```python
from build123d import *

# Parameters (mm, degrees)
EXTRUDE_1_DEPTH     = 1
EXTRUDE_2_DEPTH     = 20
CUT_EXTRUDE_1_DEPTH = 20


with BuildPart() as part:
    # 草图1 → 凸台-拉伸1 (new body)
    with BuildSketch(Plane.XY):
        with BuildLine():
            Line((0, 38), (33, 38))
            ThreePointArc((33, 38), (71, 0), (33, -38))
            Line((33, -38), (0, -38))
            ThreePointArc((0, -38), (-38, 0), (0, 38))
        make_face()
    extrude(amount=EXTRUDE_1_DEPTH)

    # 草图2 → 凸台-拉伸2 (add)
    with BuildSketch(Plane.XY.offset(1)):
        with BuildLine():
            Line((0, 38), (33, 38))
            ThreePointArc((33, 38), (71, 0), (33, -38))
            Line((33, -38), (0, -38))
            ThreePointArc((0, -38), (-38, 0), (0, 38))
        make_face()
        with BuildLine():
            Line((0, 37), (33, 37))
            ThreePointArc((33, 37), (70, 0), (33, -37))
            Line((33, -37), (0, -37))
            ThreePointArc((0, -37), (-37, 0), (0, 37))
        make_face(mode=Mode.SUBTRACT)
    extrude(amount=EXTRUDE_2_DEPTH)

    # 草图3 → 切除-拉伸1 (cut)
    with BuildSketch(Plane.XZ.offset(38)):
        Polygon((0, 16), (33, 16), (33, 21), (16.5, 21), (0, 21), align=None)
        with BuildLine():
            ThreePointArc((-7.575757576, 21), (-4.158348613, 17.938682084), (0, 16))
            Line((0, 16), (0, 21))
            Line((0, 21), (-7.575757576, 21))
        make_face()
        with BuildLine():
            Line((33, 21), (33, 16))
            ThreePointArc((33, 16), (37.158348613, 17.938682084), (40.575757576, 21))
            Line((40.575757576, 21), (33, 21))
        make_face()
    extrude(amount=-CUT_EXTRUDE_1_DEPTH, mode=Mode.SUBTRACT)


solid = part.part
```
Verification items for the finished model (mm, model axes). A direction names the side the tool comes from. Round coordinates to 2 decimals unless told otherwise and drop trailing zeros. Order: outer loops, then holes, each group sorted by start corner. A loop starts at its lowest first (then second) coordinate and runs counter-clockwise, first axis right, second up. Notation, with made-up numbers: (69, 8) - (115, 8) arc R23 ccw to (115, 46) - close; hole circle Ø1 at (-36, 20.25). An arc over 180 degrees is marked (long way). Use CSV: the item, a comma, the result in double quotes. Start each with the question number.
1) Section check B-B, the plane x = 15.5. Record the cut outline in (y, z), plus the area to 3 significant figures.
2) Section check A-A, the plane z = 9.5. Record the cut outline in (x, y), plus the area to 3 significant figures.
3) Go/stop test with flat-tipped pins: P1, Ø3, axis at x = 12, y = -21.5, coming from the +Z side; P2, Ø1, axis at x = -21.5, z = 15, coming from the +Y side; P3, Ø3, axis at y = -30, z = 18, coming from the -X side. Record where each tip stops, or that it passes through.
4) Mould release check, pull along Y, two halves, no side actions. Record for faces 4 (the cylindrical face through (37.1, -37.3, 17.9)), 5 (the cylindrical face through (69.99, 0.81, 10.86)), 6 (the flat face through (16, 38, 10)): +Y half, -Y half, draft (parallel to the pull), parting line (faces both ways), or undercut.
5) Section check C-C, the plane y = 5. Record the cut outline in (x, z), plus the area to 3 significant figures.
6) Access from +Z, -Z, +X, -X, +Y, -Y to the whole of each face (thin tool, end or side, straight path). Record for faces 1 (the cylindrical face through (-4.212, -37.319, 17.974)), 2 (the flat face through (41, 36.8, 21)), 3 (the flat face through (16, 37, 11)).
7) Thickness scan on L1, parallel to Z at x = -5.5, y = -22; L2, parallel to X at y = 27.5, z = 15.5; L3, parallel to X at y = 9, z = 11.25. Record the ranges inside material, lowest first.
Answers:
1,outline,"(-38, 0) - (38, 0) - (38, 21) - (37, 21) - (37, 1) - (-37, 1) - (-37, 16) - (-38, 16) - close"
1,area,"111 mm²"
2,outline,"(0, -38) - (33, -38) arc R38 ccw to (33, 38) - (0, 38) arc R38 ccw to start; hole (0, -37) - (33, -37) arc R37 ccw to (33, 37) - (0, 37) arc R37 ccw to start"
2,area,"302 mm²"
3,P1,"stops at z = 1"
3,P2,"stops at y = 31.67"
3,P3,"stops at x = -25.13"
4,face 4,"draft"
4,face 5,"undercut"
4,face 6,"+Y half"
5,outline,"(-37.67, 0) - (70.67, 0) - (70.67, 21) - (69.66, 21) - (69.66, 1) - (-36.66, 1) - (-36.66, 21) - (-37.67, 21) - close"
5,area,"149 mm²"
6,face 1,"+Z, -Y"
6,face 2,"+Z, +X, -X, +Y, -Y"
6,face 3,"+Z"
7,L1,"z = 0 to 1"
7,L2,"x = -26.22 to -24.75, 57.75 to 59.22"
7,L3,"x = -36.92 to -35.89, 68.89 to 69.92"
